from build123d import *

# Parameters (mm, degrees)
SKETCH1_W                    = 121.4
SKETCH1_H                    = 120.087935058
SKETCH1_R                    = 12.7
BASE_FLANGE1_DEPTH           = 3.175
EDGE_FLANGE1_STRIP_W         = 14.1732
EDGE_FLANGE1_STRIP_H         = 3.175
EDGE_FLANGE1_STRIP_CUT_DEPTH = 121.4
EDGE_FLANGE1_DEPTH           = 121.4
FILLET1_R                    = 2.54
SKETCH9_R                    = 3.205
LOWER_T_SLOT_HOLES_DEPTH     = 135.888231543
SKETCH10_R                   = 3.206253706
UPPER_T_SLOT_HOLES_DEPTH     = 92.616264341


# Sheet-metal steps are written as plain solids
with BuildPart() as part:
    # Sketch1 → Base-Flange1 (new body)
    with BuildSketch(Plane(origin=(0, 0, 0), x_dir=(0, 1, 0), z_dir=(0, 0, 1))):
        with Locations((-2.8, 2.143967529)):
            Rectangle(SKETCH1_W, SKETCH1_H)
        with Locations(Location((0, 0, 0), (0, 0, 270))):
            Circle(SKETCH1_R, mode=Mode.SUBTRACT)
    extrude(amount=BASE_FLANGE1_DEPTH)

    # Edge-Flange1 strip (across the edge) → Edge-Flange1 strip cut (cut)
    with BuildSketch(Plane(origin=(-62.187935058, -63.5, 0), x_dir=(1, 0, 0), z_dir=(0, 1, 0))):
        with Locations((-3.175, -1.5875)):
            Rectangle(EDGE_FLANGE1_STRIP_W, EDGE_FLANGE1_STRIP_H)
    extrude(amount=EDGE_FLANGE1_STRIP_CUT_DEPTH, mode=Mode.SUBTRACT)

    # Edge-Flange1 section (across the edge) → Edge-Flange1 (add)
    with BuildSketch(Plane(origin=(-62.187935058, -63.5, 0), x_dir=(1, 0, 0), z_dir=(0, 1, 0))):
        with BuildLine():
            Line((0, 0.7366), (0, 22.225))
            Line((0, 22.225), (3.175, 22.225))
            Line((3.175, 22.225), (3.175, 0.7366))
            ThreePointArc((3.175, 0.7366), (3.390745145, 0.215745145), (3.9116, 0))
            Line((3.9116, 0), (3.9116, -3.175))
            ThreePointArc((3.9116, -3.175), (1.145681115, -2.029318885), (0, 0.7366))
        make_face()
    extrude(amount=EDGE_FLANGE1_DEPTH)

    # Fillet1
    fillet1_edges = [part.edges().sort_by_distance(p)[0] for p in [
        (-60.600435058, -63.5, -22.225),
        (-60.600435058, 57.9, -22.225),
        (57.9, 57.9, 1.5875),
        (57.9, -63.5, 1.5875),
    ]]
    fillet(fillet1_edges, radius=FILLET1_R)

    # Sketch9 → Lower T-Slot Holes (cut, through all)
    with BuildSketch(Plane.YZ.offset(-59.012935058)):
        with Locations(Location((45.2, -9.525, 0), (0, 0, 270))):
            Circle(SKETCH9_R)
        with Locations(Location((-25.4, -9.525, 0), (0, 0, 270))):
            Circle(SKETCH9_R)
    extrude(amount=-LOWER_T_SLOT_HOLES_DEPTH, mode=Mode.SUBTRACT)

    # Sketch10 → Upper T-Slot Holes (cut, through all)
    with BuildSketch(Plane(origin=(0, 0, 0), x_dir=(1, 0, 0), z_dir=(0, 0, -1))):
        with Locations(Location((-45.576335058, 50.8, 0), (0, 0, 180))):
            Circle(SKETCH10_R)
        with Locations(Location((45.2, 50.8, 0), (0, 0, 180))):
            Circle(SKETCH10_R)
    extrude(amount=-UPPER_T_SLOT_HOLES_DEPTH, mode=Mode.SUBTRACT)


solid = part.part
Geometry: final body of the model. Coordinates: model frame, mm. A direction names the side the tool comes from. Give positions to 0.01 mm unless a question says otherwise; leave off trailing zeros. Loops run counter-clockwise (first coordinate to the right, second up) from the corner with the lowest first, then second, coordinate; pieces in that order, holes last. Notation, with made-up numbers: M 4.5,56.5 L 26.5,56.5 A29 cw 26.5,79.5 Z; hole C 17,14 d11. An arc over 180 degrees is marked long. Put each result on its own line as item: value.
1) Cut plane A-A, the plane x = 0. Return the cut outline in (y, z) (3 decimals), plus the area to 3 significant figures.
Computed values:
outline: M -63.5,0 L -12.7,0 L -12.7,3.175 L -63.5,3.175 Z; M 12.7,0 L 57.9,0 L 57.9,3.175 L 12.7,3.175 Z
area: 305 mm^2
2) Cut plane B-B, the plane y = -25.4. Return the cut outline in (x, z) (3 decimals), plus the area to 3 significant figures.
Computed values:
outline: M -62.188,-22.225 L -59.013,-22.225 L -59.013,-12.73 L -62.188,-12.73 Z; M -62.188,-6.32 L -59.013,-6.32 L -59.013,-0.737 A0.737 cw -58.276,0 L 57.9,0 L 57.9,3.175 L -58.276,3.175 A3.912 ccw -62.188,-0.737 Z
area: 428 mm^2
3) Cut plane C-C, the plane x = 45.2. Return the cut outline in (y, z) (3 decimals).
Computed values:
outline: M -63.5,0 L -54.006,0 L -54.006,3.175 L -63.5,3.175 Z; M -47.594,0 L 57.9,0 L 57.9,3.175 L -47.594,3.175 Z
4) First-contact query: P1, Ø12, axis at x = -48.5, y = -17, coming from the -Z side; P2, Ø10.5, axis at y = -20.5, z = -6, coming from the +X side. Flat tips, straight axial feed; report the tip coordinate or a pass-through.
Computed values:
P1: stops at z = 0
P2: stops at x = -59.01
5) Material intervals for L1, parallel to Y at x = 45.2, z = 1.45; L2, parallel to X at y = -30, z = -10.5; L3, parallel to Y at x = 0, z = 1.25, sorted ascending. Write a range as from..to.
Computed values:
L1: y = -63.5..-54.01, -47.59..57.9
L2: x = -62.19..-59.01
L3: y = -63.5..-12.7, 12.7..57.9
6) Cut plane D-D, the plane y = 32.5. Return the cut outline in (x, z) (3 decimals), plus the area to 3 significant figures.
Computed values:
outline: M -62.188,-22.225 L -59.013,-22.225 L -59.013,-0.737 A0.737 cw -58.276,0 L 57.9,0 L 57.9,3.175 L -58.276,3.175 A3.912 ccw -62.188,-0.737 Z
area: 449 mm^2
7) Mould query, pull axis X, two halves, no side actions, for faces 1 (the cylindrical face through (-10.1, -7.7, 1.6)), 2 (the cylindrical face through (-61.01, -3.65, 2.06)), 3 (the flat face through (-12, 57.9, 1)). Classes: released by +X, released by -X, zero draft, split by the parting line, or undercut.
Computed values:
face 1: undercut
face 2: released by -X
face 3: zero draft
8) Reachability of faces 4 (the cylindrical face through (-43.03, -52.75, 1.57)), 5 (the flat face through (-59.013, -4, -12)) from +Z, -Z, +X, -X, +Y, -Y: full face, straight path, thin tool, end or side. Return the list, or none.
Computed values:
face 4: +Z, -Z
face 5: -Z, +X, +Y, -Y
